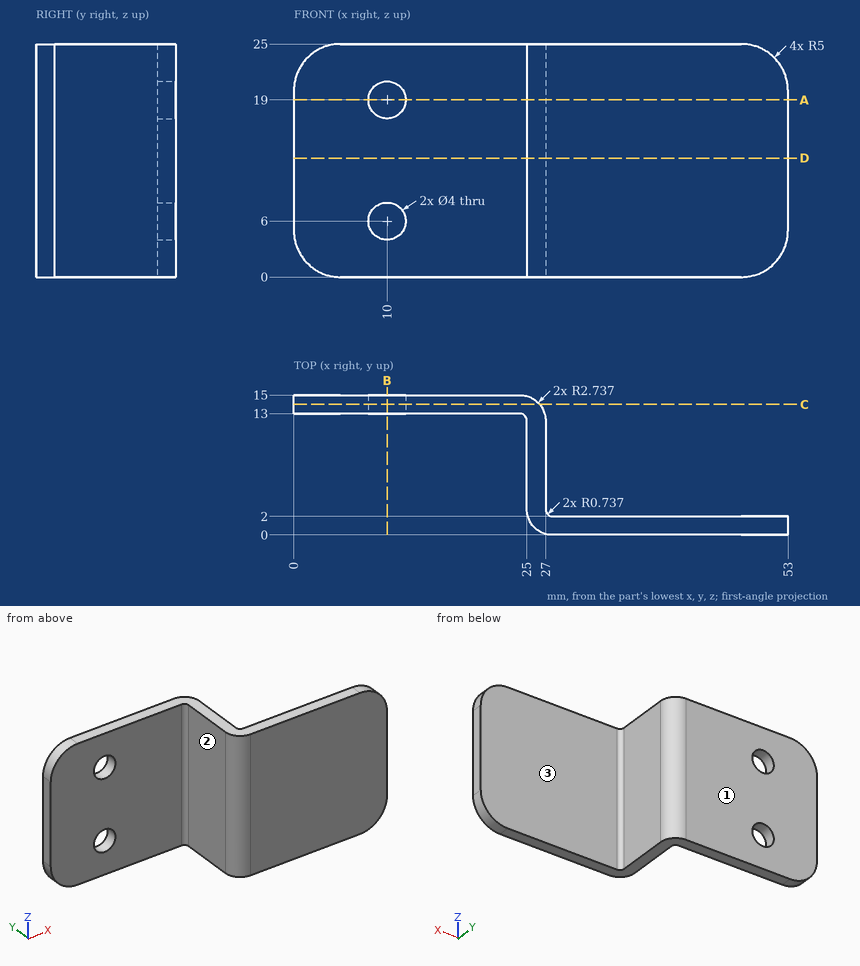
Study the drawing (mm; zero at the part's minimum x, y, z) and answer. A direction names the side the tool comes from. Coordinates: 2 decimals unless noted, no trailing zeros. Write each loop counter-clockwise with the first axis right and the second up, starting at its lowest first coordinate (ties: lowest second). Pieces come first, ordered by that corner, then holes.
Q1. Given P1, Ø1.5, axis at y = 3.5, z = 11.5, coming from the +X side; P2, Ø4, axis at y = 10.5, z = 13, coming from the -X side; P3, Ø3, axis at y = 12, z = 3.5, coming from the -X side (1 decimal), each flat-ended and moving along its own axis, determine where each tip first touches the part or whether it passes through.
Returned:
P1: stops at x = 27
P2: stops at x = 24.96
P3: stops at x = 0
Q2. Which of the six approach directions +Z, -Z, +X, -X, +Y, -Y give full straight-line access (tool end or side, diameter ignored) to the marked faces 1, 2 and 3?
Returned:
face 1: +Z, -Z, +X, -X, +Y
face 2: +Z, -Z, -X, -Y
face 3: +Z, -Z, +X, +Y
Q3. Section D-D, the plane z = 12.75 is taken. Write down the section's boundary in (x, y).
Returned:
outline: (0, 13) - (24.26, 13) arc R0.74 cw to (25, 12.26) - (25, 2.74) arc R2.74 ccw to (27.74, 0) - (53, 0) - (53, 2) - (27.74, 2) arc R0.74 cw to (27, 2.74) - (27, 12.26) arc R2.74 ccw to (24.26, 15) - (0, 15) - close
Q4. Section C-C, the plane y = 14 is taken. Write down the section's boundary in (x, z).
Returned:
outline: (0, 5) arc R5 ccw to (5, 0) - (26.38, 0) - (26.38, 25) - (5, 25) arc R5 ccw to (0, 20) - close; hole circle Ø4 at (10, 6); hole circle Ø4 at (10, 19)
Q5. Section A-A, the plane z = 19 is taken. Write down the section's boundary in (x, y).
Returned:
outline: (0, 13) - (8, 13) - (8, 15) - (0, 15) - close; (12, 13) - (24.26, 13) arc R0.74 cw to (25, 12.26) - (25, 2.74) arc R2.74 ccw to (27.74, 0) - (53, 0) - (53, 2) - (27.74, 2) arc R0.74 cw to (27, 2.74) - (27, 12.26) arc R2.74 ccw to (24.26, 15) - (12, 15) - close
Q6. Section B-B, the plane x = 10 is taken. Write down the section's boundary in (y, z).
Returned:
outline: (13, 0) - (15, 0) - (15, 4) - (13, 4) - close; (13, 8) - (15, 8) - (15, 17) - (13, 17) - close; (13, 21) - (15, 21) - (15, 25) - (13, 25) - close
Q7. Find the intervals of material crossed by line 1 along Z through (x, y) = (10, 13.95); line 2 along Y through (x, z) = (36.5, 9.75); line 3 along Y through (x, z) = (8, 21.75), in increasing order.
Returned:
line 1: z = 0 to 4, 8 to 17, 21 to 25
line 2: y = 0 to 2
line 3: y = 13 to 15
